Geometry check sheet. Reference: the model listing, model coordinates, mm. A direction names the side the tool comes from. Round coordinates to 2 decimals unless told otherwise and drop trailing zeros. Loops run counter-clockwise (first coordinate to the right, second up) from the corner with the lowest first, then second, coordinate; pieces in that order, holes last. Notation, with made-up numbers: (-4, 88) -> (44, 88) arc R19 ccw to (44, 107) -> close; hole circle Ø5 at (48.25, -4). An arc over 180 degrees is marked (long way). Use one line per item in the form item = value.
from build123d import *

# Parameters (mm, degrees)
F1_DEPTH = 8


with BuildPart() as f1:
    # F0 (on Top) → F1 (new body)
    with BuildSketch(Plane.XY):
        with BuildLine():
            Line((26, 32), (-26, 32))
            ThreePointArc((-26, 32), (-48.627417, 22.627417), (-58, 0))
            ThreePointArc((-58, 0), (-48.627417, -22.627417), (-26, -32))
            Line((-26, -32), (26, -32))
            ThreePointArc((26, -32), (48.627417, -22.627417), (58, 0))
            ThreePointArc((58, 0), (48.627417, 22.627417), (26, 32))
        make_face()
        with BuildLine():
            ThreePointArc((-49, -4), (-53, 0), (-49, 4))
            Line((-49, 4), (-41, 4))
            ThreePointArc((-41, 4), (-37, 0), (-41, -4))
            Line((-41, -4), (-49, -4))
        make_face(mode=Mode.SUBTRACT)
        with BuildLine():
            Line((49, -4), (41, -4))
            ThreePointArc((41, -4), (37, 0), (41, 4))
            Line((41, 4), (49, 4))
            ThreePointArc((49, 4), (53, 0), (49, -4))
        make_face(mode=Mode.SUBTRACT)
    extrude(amount=F1_DEPTH)


solid = f1.part
1. Gauge pin test, flat ends, axial feed: pin 1 (8 mm diameter, centred on x = -12.5, y = 12.5, fed in from -Z); pin 2 (2.5 mm diameter, centred on x = -46, z = 4, fed in from -Y); pin 3 (3 mm diameter, centred on x = -41.5, z = 5, fed in from +Y) (3 decimals); pin 4 (2 mm diameter, centred on y = 15.5, z = 6, fed in from +X). Record the tip position at first contact, or that the pin passes through.
Return value:
pin_1 = 0
pin_2 = -25.93
pin_3 = 28.775
pin_4 = 54.53
2. Section check A-A (z = 2.25). Record the boundary of the cut face in (x, y), then the cut area to 3 significant figures.
Return value:
outline = (-26, -32) -> (26, -32) arc R32 ccw to (26, 32) -> (-26, 32) arc R32 ccw to start; hole (-49, -4) -> (-41, -4) arc R4 ccw to (-41, 4) -> (-49, 4) arc R4 ccw to start; hole (41, -4) -> (49, -4) arc R4 ccw to (49, 4) -> (41, 4) arc R4 ccw to start
area = 6,320 mm2
3. Mould release check, pull along X, two halves, no side actions. Record for faces 1 (the flat face through (0, -32, 4)), 2 (the cylindrical face through (53, 0, 4)): released by +X, released by -X, zero draft, split by the parting line, or undercut.
Return value:
face_1 = zero draft
face_2 = undercut
4. Material ranges on line 1 along X through (y, z) = (1, 2.75); line 2 along Y through (x, z) = (-51, 3); line 3 along Y through (x, z) = (49.5, 2.25), recorded low to high.
Return value:
line_1 = -57.98 to -52.87, -37.13 to 37.13, 52.87 to 57.98
line_2 = -19.97 to -3.46, 3.46 to 19.97
line_3 = -21.72 to -3.97, 3.97 to 21.72
5. Tool access check on faces 3 (the cylindrical face through (-53, 0, 4)), 4 (the flat face through (-1, 0, 8)). Record the directions out of +Z, -Z, +X, -X, +Y, -Y that give a thin tool (end or side, any length) a straight path to the whole face; none if there is none.
Return value:
face_3 = +Z, -Z
face_4 = +Z, +X, -X, +Y, -Y
6. Section check C-C (y = 23). Record the boundary of the cut face in (x, z).
Return value:
outline = (-48.25, 0) -> (48.25, 0) -> (48.25, 8) -> (-48.25, 8) -> close
7. Section check D-D (y = -25). Record the boundary of the cut face in (x, z).
Return value:
outline = (-45.97, 0) -> (45.97, 0) -> (45.97, 8) -> (-45.97, 8) -> close
8. Section check B-B (x = 45). Record the boundary of the cut face in (y, z), then the cut area to 3 significant figures.
Return value:
outline = (-25.75, 0) -> (-4, 0) -> (-4, 8) -> (-25.75, 8) -> close; (4, 0) -> (25.75, 0) -> (25.75, 8) -> (4, 8) -> close
area = 348 mm2
